from build123d import *

# Parameters (mm, degrees)
F1_DEPTH = 5
F3_D     = 4
F4_W     = 5.6
F4_H     = 21
F5_DEPTH = 5


with BuildPart() as f1:
    # F0 (on Top) → F1 (new body)
    with BuildSketch(Plane.XY):
        Polygon((52.2, 31.5), (52.2, 52.5), (-57.8, 52.5), (-57.8, -52.5), (52.2, -52.5), (52.2, -31.5), (57.8, -31.5), (57.8, -10.5), (52.2, -10.5), (52.2, 10.5), (57.8, 10.5), (57.8, 31.5), align=None)
    extrude(amount=F1_DEPTH)

    # F3 (through all)
    with Locations(Plane.XZ.offset(31.5)):
        with Locations((54.670613, 2.486458)):
            Hole(F3_D / 2)

    # F4 (on face) → F5 (join)
    with BuildSketch(Plane.XY.offset(5)):
        with Locations((55, 21)):
            Rectangle(F4_W, F4_H)
        with Locations((55, -21)):
            Rectangle(F4_W, F4_H)
    extrude(amount=F5_DEPTH)


solid = f1.part
Work out the finished part from the listing and answer in its coordinate system (mm). A direction names the side the tool comes from. Round coordinates to 2 decimals unless told otherwise and drop trailing zeros. Loops run counter-clockwise (first coordinate to the right, second up) from the corner with the lowest first, then second, coordinate; pieces in that order, holes last. Notation, with made-up numbers: M 81,-8 L 104,-8 A28 ccw 104,15 Z; hole C 88,11.5 d8. An arc over 180 degrees is marked long. One line per question, with ' | ' between items. Start each with the question number.
(1) A cutting plane is placed at B-B on y = -22.5. Write down the section's boundary in (x, z), plus the area to 3 significant figures.
(2) A cutting plane is placed at D-D on y = -39.5. Write down the section's boundary in (x, z).
(3) A cutting plane is placed at A-A on z = 7.5. Write down the section's boundary in (x, y), plus the area to 3 significant figures.
(4) For a pull along X with two mould halves and no side action, classify faces 5 (the face through (52.823, 21.147, 1.72)), 6 (the face through (-4, 1, 5)), 7 (the face through (52.2, 21, 7)) as released by +X, released by -X, zero draft, split by the parting line, or undercut.
(5) A cutting plane is placed at C-C on x = -17. Write down the section's boundary in (y, z), plus the area to 3 significant figures.
(6) A tool of negligible diameter and unlimited length cuts with its end or side. For faces 1 (the face through (52.2, 42, 2)), 2 (the face through (55, -31.5, 6)), 3 (the face through (55, 10.5, 6)), 4 (the face through (52.2, -21, 7)), from which of +Z, -Z, +X, -X, +Y, -Y can it reach the whole face along a straight path? Write none if from no direction.
(7) Flat-ended cylindrical pins translate along their axes: pin 1 Ø5 at (x, y) = (4, 1) entering from +Z; pin 2 Ø1.5 at (y, z) = (-21.5, 6.5) entering from -X; pin 3 Ø5 at (y, z) = (-5, 1.5) entering from +X; pin 4 Ø1.5 at (x, z) = (-15.5, 6.5) entering from -Y. Find the tip coordinate at first contact, or state that the pin passes through.
(8) Find the intervals of material crossed by line 1 (Y direction, x = 53, z = 5.25); line 2 (X direction, y = -29.5, z = 8); line 3 (X direction, y = 37.5, z = 3), in increasing order.
Geometry check:
1) outline: M -57.8,0 L 57.8,0 L 57.8,10 L 52.2,10 L 52.2,5 L -57.8,5 Z; hole C 54.67,2.49 d4 | area: 593 mm²
2) outline: M -57.8,0 L 52.2,0 L 52.2,5 L -57.8,5 Z
3) outline: M 52.2,-31.5 L 57.8,-31.5 L 57.8,-10.5 L 52.2,-10.5 Z; M 52.2,10.5 L 57.8,10.5 L 57.8,31.5 L 52.2,31.5 Z | area: 235 mm²
4) face 5: undercut | face 6: zero draft | face 7: released by -X
5) outline: M -52.5,0 L 52.5,0 L 52.5,5 L -52.5,5 Z | area: 525 mm²
6) face 1: +Z, -Z, +X, +Y | face 2: +Z, -Z, +X, -Y | face 3: +Z, -Z, +X | face 4: +Z, -X, +Y, -Y
7) pin 1: stops at z = 5 | pin 2: stops at x = 52.2 | pin 3: stops at x = 52.2 | pin 4: passes through
8) line 1: y = -31.5 to -10.5, 10.5 to 31.5 | line 2: x = 52.2 to 57.8 | line 3: x = -57.8 to 52.2
